Here's how the part is built. I have some questions about the finished solid (model axes, mm). Face numbers are marked on the shaded views. A direction names the side the tool comes from. Round coordinates to 2 decimals unless told otherwise and drop trailing zeros. Write each loop counter-clockwise with the first axis right and the second up, starting at its lowest first coordinate (ties: lowest second). Pieces come first, ordered by that corner, then holes. Notation, with made-up numbers: (9.25, 10) -> (20.25, 10) arc R6 cw to (20.25, 17) -> close; hole circle Ø5 at (-38, 13.25). An arc over 180 degrees is marked (long way). Answer as CSV lines item,"result".
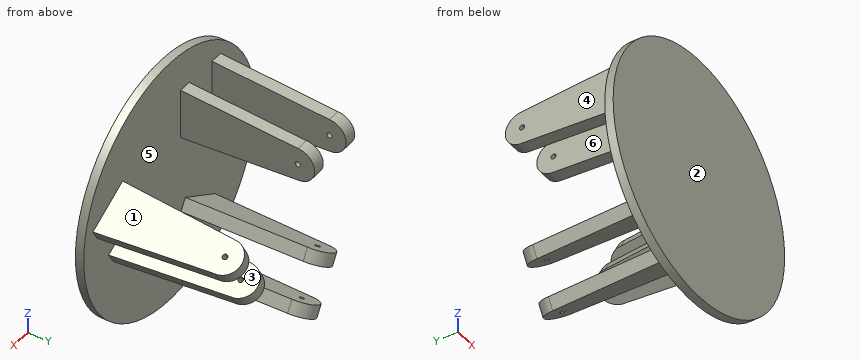
```python
from build123d import *

# Parameters (mm, degrees)
SKETCH2_R          = 75
EXTRUDE1_DEPTH     = 5
EXTRUDE3_START     = 5
SKETCH1_W          = 7.5
SKETCH1_H          = 30
EXTRUDE3_DEPTH     = 80
SKETCH3_R          = 1.5
CUT_EXTRUDE1_DEPTH = 55
CIRPATTERN1_COUNT  = 3


with BuildPart() as part:
    # Sketch2 → Extrude1 (new body)
    with BuildSketch(Plane(origin=(0, 0, 0), x_dir=(1, 0, 0), z_dir=(0, 1, 0))):
        with Locations(Location((0, 0, 0), (0, 0, 270))):
            Circle(SKETCH2_R)
    extrude(amount=EXTRUDE1_DEPTH)

    # Sketch1 → Extrude3 (add)
    with BuildSketch(Plane(origin=(0, 0, 0), x_dir=(1, 0, 0), z_dir=(0, 1, 0)).offset(EXTRUDE3_START)):
        with Locations((-13.439285714, -36.554084254)):
            Rectangle(SKETCH1_W, SKETCH1_H)
        with Locations((-40.939285714, -36.554084254)):
            Rectangle(SKETCH1_W, SKETCH1_H)
    extrude3 = extrude(amount=EXTRUDE3_DEPTH)

    # Sketch3 → Cut-Extrude1 (cut)
    with BuildSketch(Plane(origin=(0, 0, 0), x_dir=(0, 0, -1), z_dir=(1, 0, 0))):
        with Locations((-36.554084254, 75)):
            Circle(SKETCH3_R)
        with BuildLine():
            Line((-51.554084254, 5), (-52.554084254, 6))
            Line((-52.554084254, 6), (-52.554084254, 86))
            Line((-52.554084254, 86), (-20.554084254, 86))
            Line((-20.554084254, 86), (-20.554084254, 6))
            Line((-20.554084254, 6), (-21.554084254, 5))
            Line((-21.554084254, 5), (-26.554084254, 75))
            ThreePointArc((-26.554084254, 75), (-36.554084254, 85), (-46.554084254, 75))
            Line((-46.554084254, 75), (-51.554084254, 5))
        make_face()
    cut_extrude1 = extrude(amount=-CUT_EXTRUDE1_DEPTH, mode=Mode.SUBTRACT)

    # CirPattern1: Extrude3, Cut-Extrude1 ×3 about axis
    cirpattern1_axis = Axis((0, 0, 0), (0, 1, 0))
    add([extrude3.rotate(cirpattern1_axis, i * 360 / CIRPATTERN1_COUNT) for i in range(1, CIRPATTERN1_COUNT)])
    add([cut_extrude1.rotate(cirpattern1_axis, i * 360 / CIRPATTERN1_COUNT) for i in range(1, CIRPATTERN1_COUNT)], mode=Mode.SUBTRACT)


solid = part.part
```
1. If we mould it in two halves opening along Z, with no side actions, what happens to the marked faces 1, 2 and 3? For each: released by +Z, released by -Z, zero draft, split by the parting line, or undercut.
Numbers:
face 1,"released by +Z"
face 2,"zero draft"
face 3,"undercut"
2. If I drill on line 1 (Z direction, x = -12, y = 75); line 2 (X direction, y = 36.5, z = 44); line 3 (Y direction, x = -43, z = -12), over which ranges is the centre line in solid material (lowest first)?
Numbers:
line 1,"z = -58.53 to -55.32, 26.55 to 35.05, 38.05 to 46.55"
line 2,"x = -44.69 to -37.19, -17.19 to -9.69"
line 3,"y = 0 to 5"
3. On a 3-axis mill with a long thin cutter (end or side, diameter ignored), from which of +Z, -Z, +X, -X, +Y, -Y can I reach the whole of each face in a straight line? I mean the marked faces 4, 5 and 6. Say none if no direction works.
Numbers:
face 4,"+Z, -Z, -X, +Y"
face 5,"+Y"
face 6,"+Z, +Y"
4. For pin 1 Ø24 at (y, z) = (44, 41.5) entering from -X; pin 2 Ø1.5 at (x, y) = (-11.5, 20) entering from -Z; pin 3 Ø15 at (y, z) = (30.5, 39.5) entering from +X; pin 4 Ø2.5 at (y, z) = (75, 36.55) entering from -X, each with a flat end and sliding along its axis, tell me the tip position at first contact or that it passes through.
Numbers:
pin 1,"stops at x = -44.69"
pin 2,"stops at z = -58.68"
pin 3,"stops at x = -9.69"
pin 4,"passes through"
5. Suppose I cut it at A-A on y = 64.5. Please give me the cut outline in (x, z).
Numbers:
outline,"(-44.69, 25.8) -> (-37.19, 25.8) -> (-37.19, 47.3) -> (-44.69, 47.3) -> close; (-36.12, -32.04) -> (-32.37, -38.54) -> (-13.75, -27.79) -> (-17.5, -21.29) -> close; (-22.37, -55.86) -> (-18.62, -62.35) -> (0, -51.6) -> (-3.75, -45.11) -> close; (-17.19, 25.8) -> (-9.69, 25.8) -> (-9.69, 47.3) -> (-17.19, 47.3) -> close; (27.19, -4.51) -> (45.81, -15.26) -> (49.56, -8.77) -> (30.94, 1.98) -> close; (40.94, 19.3) -> (59.56, 8.55) -> (63.31, 15.05) -> (44.69, 25.8) -> close"
6. Suppose I cut it at B-B on y = 26. Please give me the cut outline in (x, z), and give its area (4 significant figures).
Numbers:
outline,"(-44.69, 23.05) -> (-37.19, 23.05) -> (-37.19, 50.05) -> (-44.69, 50.05) -> close; (-38.5, -33.42) -> (-34.75, -39.91) -> (-11.37, -26.41) -> (-15.12, -19.92) -> close; (-24.75, -57.23) -> (-21, -63.73) -> (2.38, -50.23) -> (-1.37, -43.73) -> close; (-17.19, 23.05) -> (-9.69, 23.05) -> (-9.69, 50.05) -> (-17.19, 50.05) -> close; (24.81, -3.14) -> (48.19, -16.64) -> (51.94, -10.14) -> (28.56, 3.36) -> close; (38.56, 20.68) -> (61.94, 7.18) -> (65.69, 13.68) -> (42.31, 27.18) -> close"
area,"1,215 mm^2"
